Input: part model. Units: mm. Frame: model coordinates. A direction names the side the tool comes from. Give positions to 0.01 mm unless a question says otherwise; leave off trailing zeros. Loops run counter-clockwise (first coordinate to the right, second up) from the corner with the lowest first, then second, coordinate; pieces in that order, holes last. Notation, with made-up numbers: (12, 13.5) -> (60, 13.5) arc R14 cw to (60, 20.5) -> close; hole circle Ø2 at (63.25, 12). An arc over 180 degrees is marked (long way). Answer as a JSON object with one key per item and string values.
```python
from build123d import *

# Parameters (mm, degrees)
SKETCH_1_W          = 60
SKETCH_1_H          = 30
SKETCH_1_R          = 2
SKETCH_1_R_2        = 1.75
EXTRUDE_1_DEPTH     = 14
FILLET_1_R          = 10
SKETCH_2_R          = 3.5
CUT_EXTRUDE_1_DEPTH = 4.5


with BuildPart() as part:
    # 草图1 → 凸台-拉伸1 (new body)
    with BuildSketch(Plane(origin=(0, 0, 0), x_dir=(1, 0, 0), z_dir=(0, 1, 0))):
        Rectangle(SKETCH_1_W, SKETCH_1_H)
        with Locations(Location((-20, 0, 0), (0, 0, 270))):
            Circle(SKETCH_1_R, mode=Mode.SUBTRACT)
        with Locations(Location((-20, 10, 0), (0, 0, 270))):
            Circle(SKETCH_1_R_2, mode=Mode.SUBTRACT)
        with Locations(Location((20, 10, 0), (0, 0, 270))):
            Circle(SKETCH_1_R_2, mode=Mode.SUBTRACT)
        with Locations(Location((-20, -10, 0), (0, 0, 270))):
            Circle(SKETCH_1_R_2, mode=Mode.SUBTRACT)
        with Locations(Location((20, -10, 0), (0, 0, 270))):
            Circle(SKETCH_1_R_2, mode=Mode.SUBTRACT)
    extrude(amount=EXTRUDE_1_DEPTH)

    # 圆角1
    fillet_1_edges = [part.edges().sort_by_distance(p)[0] for p in [
        (-30, 7, 15),
        (-30, 7, -15),
    ]]
    fillet(fillet_1_edges, radius=FILLET_1_R)

    # 草图2 → 切除-拉伸1 (cut)
    with BuildSketch(Plane(origin=(0, 14, 0), x_dir=(1, 0, 0), z_dir=(0, 1, 0))):
        with Locations(Location((-20, 10, 0), (0, 0, 270))):
            Circle(SKETCH_2_R)
        with Locations(Location((-20, -10, 0), (0, 0, 270))):
            Circle(SKETCH_2_R)
        with Locations(Location((20, 10, 0), (0, 0, 270))):
            Circle(SKETCH_2_R)
        with Locations(Location((20, -10, 0), (0, 0, 270))):
            Circle(SKETCH_2_R)
    extrude(amount=-CUT_EXTRUDE_1_DEPTH, mode=Mode.SUBTRACT)


solid = part.part
```
Q1. Section B-B, the plane x = 20. Return the cut outline in (y, z).
Evaluation:
{"outline": "(0, -15) -> (14, -15) -> (14, -13.5) -> (9.5, -13.5) -> (9.5, -11.75) -> (0, -11.75) -> close; (0, -8.25) -> (9.5, -8.25) -> (9.5, -6.5) -> (14, -6.5) -> (14, 6.5) -> (9.5, 6.5) -> (9.5, 8.25) -> (0, 8.25) -> close; (0, 11.75) -> (9.5, 11.75) -> (9.5, 13.5) -> (14, 13.5) -> (14, 15) -> (0, 15) -> close"}
Q2. Section A-A, the plane z = 0. Return the cut outline in (x, y).
Evaluation:
{"outline": "(-30, 0) -> (-22, 0) -> (-22, 14) -> (-30, 14) -> close; (-18, 0) -> (30, 0) -> (30, 14) -> (-18, 14) -> close"}
Q3. Pin query (flat end, axial travel): pin 1 (5.5 mm diameter, centred on x = 20.5, z = 9.5, fed in from +Y). Return the tip coordinate at first contact, or that it passes through.
Evaluation:
{"pin 1": "stops at y = 9.5"}
Q4. Section C-C, the plane y = 7.25. Return the cut outline in (x, z).
Evaluation:
{"outline": "(-30, -5) arc R10 ccw to (-20, -15) -> (30, -15) -> (30, 15) -> (-20, 15) arc R10 ccw to (-30, 5) -> close; hole circle Ø4 at (-20, 0); hole circle Ø3.5 at (-20, -10); hole circle Ø3.5 at (-20, 10); hole circle Ø3.5 at (20, -10); hole circle Ø3.5 at (20, 10)"}
Q5. Ray query, line 1 along Z through (x, y) = (20, 6.5); line 2 along X through (y, z) = (7, -10.5); line 3 along X through (y, z) = (12.65, 10). Return the intervals inside material, ascending.
Evaluation:
{"line 1": "z = -15 to -11.75, -8.25 to 8.25, 11.75 to 15", "line 2": "x = -28.35 to -21.68, -18.32 to 18.32, 21.68 to 30", "line 3": "x = -28.66 to -23.5, -16.5 to 16.5, 23.5 to 30"}
Q6. Access query for faces 1 (the cylindrical face through (-17.635, 11.782, 7.42)), 2 (the cylindrical face through (-18.265, 4.684, -10.228)). Directions: +Z, -Z, +X, -X, +Y, -Y. A direction counts if a zero-diameter tool reaches every point of the face in a straight line with its end or side. Return the directions, or none.
Evaluation:
{"face 1": "+Y", "face 2": "+Y, -Y"}
Q7. Draft query along Z for faces 3 (the flat face through (5, 7, 15)), 4 (the flat face through (-18, 9.5, 11)), 5 (the flat face through (30, 7, 0)), 6 (the flat face through (5, 7, -15)). Return one class per face: +Z half, -Z half, draft (parallel to the pull), parting line (faces both ways), or undercut.
Evaluation:
{"face 3": "+Z half", "face 4": "undercut", "face 5": "draft", "face 6": "-Z half"}
Q8. Section D-D, the plane z = -10. Return the cut outline in (x, y), then the cut area to 3 significant figures.
Evaluation:
{"outline": "(-28.66, 0) -> (-21.75, 0) -> (-21.75, 9.5) -> (-23.5, 9.5) -> (-23.5, 14) -> (-28.66, 14) -> close; (-18.25, 0) -> (18.25, 0) -> (18.25, 9.5) -> (16.5, 9.5) -> (16.5, 14) -> (-16.5, 14) -> (-16.5, 9.5) -> (-18.25, 9.5) -> close; (21.75, 0) -> (30, 0) -> (30, 14) -> (23.5, 14) -> (23.5, 9.5) -> (21.75, 9.5) -> close", "area": "692 mm2"}
